```python
from build123d import *

# Parameters (mm, degrees)
DODANIE_WYCI_GNI_CIE1_DEPTH = 40
SZKIC2_W                    = 30
SZKIC2_H                    = 35
WYTNIJ_WYCI_GNI_CIE1_DEPTH  = 40
SZKIC3_R                    = 5
WYTNIJ_WYCI_GNI_CIE2_DEPTH  = 40
ZAOKR_GLENIE1_R             = 10
SZKIC4_R                    = 8
DODANIE_WYCI_GNI_CIE2_DEPTH = 30


with BuildPart() as part:
    # Szkic1 → Dodanie-wyciągnięcie1 (new body)
    with BuildSketch(Plane.XY):
        Polygon((-8.990228013, 22.917176047), (31.009771987, 22.917176047), (31.009771987, -17.082823953), (14.732595321, -17.082823953), (-8.990228013, 13.105888901), align=None)
    extrude(amount=DODANIE_WYCI_GNI_CIE1_DEPTH)

    # Szkic2 → Wytnij-wyciągnięcie1 (cut)
    with BuildSketch(Plane(origin=(31.009771987, 0, 0), x_dir=(0, 0, -1), z_dir=(1, 0, 0))):
        with Locations((-20, 0.417176047)):
            Rectangle(SZKIC2_W, SZKIC2_H)
    extrude(amount=-WYTNIJ_WYCI_GNI_CIE1_DEPTH, mode=Mode.SUBTRACT)

    # Szkic3 → Wytnij-wyciągnięcie2 (cut)
    with BuildSketch(Plane(origin=(0, 0, 0), x_dir=(-1, 0, 0), z_dir=(0, 0, -1))):
        with Locations((-11.009771987, -2.082823953)):
            Circle(SZKIC3_R)
    extrude(amount=-WYTNIJ_WYCI_GNI_CIE2_DEPTH, mode=Mode.SUBTRACT)

    # Zaokrąglenie1
    zaokr_glenie1_edges = [part.edges().sort_by_distance(p)[0] for p in [
        (31.009771987, -17.082823953, 2.5),
        (14.732595321, -17.082823953, 2.5),
        (-8.990228013, 13.105888901, 2.5),
        (31.009771987, -17.082823953, 37.5),
        (14.732595321, -17.082823953, 37.5),
        (-8.990228013, 13.105888901, 37.5),
    ]]
    fillet(zaokr_glenie1_edges, radius=ZAOKR_GLENIE1_R)

    # Szkic4 → Dodanie-wyciągnięcie2 (add)
    with BuildSketch(Plane(origin=(0, 22.917176047, 0), x_dir=(1, 0, 0), z_dir=(0, 1, 0))):
        with Locations((11.009771987, -20)):
            Circle(SZKIC4_R)
    extrude(amount=DODANIE_WYCI_GNI_CIE2_DEPTH)


solid = part.part
```
Can you work these out from the model? Positions are in its coordinate system, mm. A direction names the side the tool comes from. Give positions to 0.01 mm unless a question says otherwise; leave off trailing zeros. Loops run counter-clockwise (first coordinate to the right, second up) from the corner with the lowest first, then second, coordinate; pieces in that order, holes last. Notation, with made-up numbers: M 22,-7 L 40,-7 A18 cw 40,12 Z; hole C -23,67 d8. An arc over 180 degrees is marked long. One line per item, written item: value.
(1) Suppose I cut it at A-A on z = 20. List the corners of the cut face in (x, y) for me.
Returned:
outline: M -8.99,17.92 L 31.01,17.92 L 31.01,22.92 L 19.01,22.92 L 19.01,52.92 L 3.01,52.92 L 3.01,22.92 L -8.99,22.92 Z
(2) Will these pins go through, and if not, where does the flat tip stop? pin 1 (12 mm diameter, centred on x = 5.5, y = 23.5, fed in from -Z); pin 2 (2 mm diameter, centred on x = 25.5, z = 23, fed in from -Y); pin 3 (6 mm diameter, centred on y = 36, z = 11, fed in from +X); pin 4 (8 mm diameter, centred on y = 1, z = 35, fed in from -X).
Returned:
pin 1: z = 0
pin 2: y = 17.92
pin 3: x = 16.3
pin 4: x = -2.62
(3) I need wall thicknesses on line 1 (Z direction, x = 17.5, y = 3); line 2 (Y direction, x = 24, z = 8.5); line 3 (Y direction, x = 18.5, z = 22). Which ranges of each line are inside material? Lowest first, please.
Returned:
line 1: 0 to 5, 35 to 40
line 2: 17.92 to 22.92
line 3: 17.92 to 52.92
(4) Which directions (+Z, -Z, +X, -X, +Y, -Y) give clear straight access to the entire face, cutting with the end or side of a thin tool? Please do faces 4 (the face through (14.7, 37.7, 27.1)), 5 (the face through (-8.456, 13.34, 2.535)), 6 (the face through (16, 4, 35)).
Returned:
face 4: +Y
face 5: +Z, -Z, -X, -Y
face 6: +X, -X, -Y
(5) We'd pull the mould along Y, two halves only. Please class faces 1 (the face through (6.24, -0.58, 37.47)), 2 (the face through (28.158, -14.076, 2.535)), 3 (the face through (16, 8, 0)): released by +Y, released by -Y, zero draft, split by the parting line, or undercut.
Returned:
face 1: undercut
face 2: released by -Y
face 3: zero draft
(6) Suppose I cut it at C-C on y = 46.5. List the corners of the cut face in (x, z) for me.
Returned:
outline: C 11.01,20 d16
(7) Suppose I cut it at D-D on x = 17.5. List the corners of the cut face in (y, z) for me.
Returned:
outline: M -16.86,0 L 22.92,0 L 22.92,15.32 L 52.92,15.32 L 52.92,24.68 L 22.92,24.68 L 22.92,40 L -16.86,40 L -16.86,35 L 17.92,35 L 17.92,5 L -16.86,5 Z
(8) Suppose I cut it at B-B on x = 0.5. List the corners of the cut face in (y, z) for me.
Returned:
outline: M 1.03,0 L 22.92,0 L 22.92,40 L 1.03,40 L 1.03,35 L 17.92,35 L 17.92,5 L 1.03,5 Z
